```python
from build123d import *
from build123d.topology import SkipClean

# Parameters (mm, degrees)
EXTRUDE_2_DEPTH        = 8
SKETCH_5_W             = 850
SKETCH_5_H             = 100
EXTRUDE_3_DEPTH        = 8
SKETCH_6_W             = 850
SKETCH_6_H             = 8
EXTRUDE_4_DEPTH        = 84
SKETCH_7_R             = 13
CUT_EXTRUDE_1_DEPTH    = 905.579460302
SKETCH_9_R             = 13
CUT_EXTRUDE_3_DEPTH    = 904.800863022
PATTERN_LINEAR_2_COUNT = 6
PATTERN_LINEAR_2_PITCH = 160
MIRROR_7_DEPTH         = 16
MIRROR_7_2_OUTLINE_R   = 13
MIRROR_7_2_DEPTH       = 8
MIRROR_START           = 8
MIRROR_7_3_OUTLINE_R   = 13
MIRROR_7_3_DEPTH       = 8
MIRROR_START_2         = 16
MIRROR_7_4_OUTLINE_W   = 850
MIRROR_7_4_OUTLINE_H   = 8
MIRROR_7_4_DEPTH       = 84


# Read off the part's stored shape, not the designer's step: 镜向7
with BuildPart() as part:
    # 草图1 → 凸台-拉伸2 (new body)
    with BuildSketch(Plane.XY):
        Polygon((-870, 0), (-870, 230), (-770, 230), (0, 100), (0, 0), align=None)
    extrude_2 = extrude(amount=EXTRUDE_2_DEPTH)

    # 镜向2: 凸台-拉伸2 across plane
    add(extrude_2.mirror(Plane.ZX))

    # 草图5 → 凸台-拉伸3 (add)
    with BuildSketch(Plane.XY.offset(8)):
        with Locations((-425, 10)):
            Rectangle(SKETCH_5_W, SKETCH_5_H)
    extrude(amount=EXTRUDE_3_DEPTH)

    # 草图6 → 凸台-拉伸4 (add)
    with BuildSketch(Plane.XY.offset(16)):
        with Locations((-425, 56)):
            Rectangle(SKETCH_6_W, SKETCH_6_H)
    extrude(amount=EXTRUDE_4_DEPTH)

    # 草图7 → 切除-拉伸1 (cut, through all)
    with BuildSketch(Plane.XY.offset(8)):
        with Locations((-770.885465198, 130.885465198)):
            Circle(SKETCH_7_R)
        with Locations((-827.454007693, 187.454007693)):
            Circle(SKETCH_7_R)
    cut_extrude_1 = extrude(amount=-CUT_EXTRUDE_1_DEPTH, mode=Mode.SUBTRACT)

    # 镜向5: 切除-拉伸1 across plane
    add(cut_extrude_1.mirror(Plane.ZX), mode=Mode.SUBTRACT)

    # 草图9 → 切除-拉伸3 (cut, through all)
    with BuildSketch(Plane.XY.offset(16)):
        with Locations((-799.964208957, 0)):
            Circle(SKETCH_9_R)
    cut_extrude_3 = extrude(amount=-CUT_EXTRUDE_3_DEPTH, mode=Mode.SUBTRACT)

    # 阵列(线性)2: 切除-拉伸3 ×6
    with Locations(*[(i * PATTERN_LINEAR_2_PITCH, 0, 0) for i in range(1, PATTERN_LINEAR_2_COUNT)]):
        add(cut_extrude_3, mode=Mode.SUBTRACT)

    # 镜向7 outline → 镜向7 (cut)
    with BuildSketch(Plane.XY):
        with BuildLine():
            ThreePointArc((0, -12.999950731), (-12.964208957, 0), (0, 12.999950731))
            ThreePointArc((0, 12.999950731), (-13.035791043, 0), (0, -12.999950731))
        make_face()
    extrude(amount=MIRROR_7_DEPTH, mode=Mode.SUBTRACT)

    # Mirror 7 2 outline → Mirror 7 2 (add)
    with BuildSketch(Plane.XY):
        with BuildLine():
            Line((870, -230), (870, 230))
            Line((870, 230), (770, 230))
            Line((770, 230), (0, 100))
            Line((0, 100), (0, 12.999950731))
            ThreePointArc((0, 12.999950731), (12.964208957, 0), (0, -12.999950731))
            Line((0, -12.999950731), (0, -100))
            Line((0, -100), (770, -230))
            Line((770, -230), (870, -230))
        make_face()
        with Locations((827.454007693, -187.454007693)):
            Circle(MIRROR_7_2_OUTLINE_R, mode=Mode.SUBTRACT)
        with Locations((770.885465198, -130.885465198)):
            Circle(MIRROR_7_2_OUTLINE_R, mode=Mode.SUBTRACT)
        with Locations((770.885465198, 130.885465198)):
            Circle(MIRROR_7_2_OUTLINE_R, mode=Mode.SUBTRACT)
        with Locations((827.454007693, 187.454007693)):
            Circle(MIRROR_7_2_OUTLINE_R, mode=Mode.SUBTRACT)
        with Locations((639.964208957, 0)):
            Circle(MIRROR_7_2_OUTLINE_R, mode=Mode.SUBTRACT)
        with Locations((799.964208957, 0)):
            Circle(MIRROR_7_2_OUTLINE_R, mode=Mode.SUBTRACT)
        with Locations((159.964208957, 0)):
            Circle(MIRROR_7_2_OUTLINE_R, mode=Mode.SUBTRACT)
        with Locations((319.964208957, 0)):
            Circle(MIRROR_7_2_OUTLINE_R, mode=Mode.SUBTRACT)
        with Locations((479.964208957, 0)):
            Circle(MIRROR_7_2_OUTLINE_R, mode=Mode.SUBTRACT)
    extrude(amount=MIRROR_7_2_DEPTH)

    # Mirror 7 3 outline → Mirror 7 3 (add)
    with SkipClean():  # the faces are left unmerged after this step: merging them gives an invalid solid
        with BuildSketch(Plane.XY.offset(MIRROR_START)):
            with BuildLine():
                Line((850, 60), (0, 60))
                Line((0, 60), (0, 12.999950731))
                ThreePointArc((0, 12.999950731), (12.964208957, 0), (0, -12.999950731))
                Line((0, -12.999950731), (0, -40))
                Line((0, -40), (850, -40))
                Line((850, -40), (850, 60))
            make_face()
            with Locations((799.964208957, 0)):
                Circle(MIRROR_7_3_OUTLINE_R, mode=Mode.SUBTRACT)
            with Locations((159.964208957, 0)):
                Circle(MIRROR_7_3_OUTLINE_R, mode=Mode.SUBTRACT)
            with Locations((319.964208957, 0)):
                Circle(MIRROR_7_3_OUTLINE_R, mode=Mode.SUBTRACT)
            with Locations((479.964208957, 0)):
                Circle(MIRROR_7_3_OUTLINE_R, mode=Mode.SUBTRACT)
            with Locations((639.964208957, 0)):
                Circle(MIRROR_7_3_OUTLINE_R, mode=Mode.SUBTRACT)
        extrude(amount=MIRROR_7_3_DEPTH)

    # Mirror 7 4 outline → Mirror 7 4 (add)
    with SkipClean():  # the faces are left unmerged after this step: merging them gives an invalid solid
        with BuildSketch(Plane.XY.offset(MIRROR_START_2)):
            with Locations((425, 56)):
                Rectangle(MIRROR_7_4_OUTLINE_W, MIRROR_7_4_OUTLINE_H)
        extrude(amount=MIRROR_7_4_DEPTH)


solid = part.part
```
Design review of the part built by this model. Coordinates are the model's own, in mm. A direction names the side the tool comes from. Coordinates: 2 decimals unless noted, no trailing zeros. Order: outer loops, then holes, each group sorted by start corner. A loop starts at its lowest first (then second) coordinate and runs counter-clockwise, first axis right, second up. Notation, with made-up numbers: M -33,18.25 L 23,18.25 A17 cw 23,41.25 Z; hole C 28.25,-23 d2. An arc over 180 degrees is marked long. Answer as a JSON object with one key per item and string values. Group by question number.
1) Add section B-B, the plane x = -198.5. Write out the cut boundary in (y, z).
2) Add section C-C, the plane z = 72.5. Write out the cut boundary in (x, y).
3) Wall thickness on L1, parallel to Z at x = -798.5, y = -142; L2, parallel to Y at x = -574, z = 56.5; L3, parallel to Z at x = 269.5, y = 9.5: over which ranges is each line inside the solid? List them lowest first.
4) For pin 1 (10 mm diameter, centred on x = 24.5, z = 62.5, fed in from -Y); pin 2 (1.5 mm diameter, centred on x = 550, y = -92.5, fed in from +Z), all flat-tipped, find the tip position at first contact; note any pin that passes through.
5) Add section A-A, the plane y = 34.5. Write out the cut boundary in (x, z).
6) Tool access review of faces 1 (the flat face through (-12, 52, 57)), 2 (the flat face through (-390.39, 165.91, 3.94)), 3 (the flat face through (379.61, -164.09, 3.94)): name each direction out of +Z, -Z, +X, -X, +Y, -Y from which nothing blocks a thin tool from reaching the whole face with its end or side.
Computed values:
{
 "1": {"outline": "M -133.51,0 L 133.51,0 L 133.51,8 L 60,8 L 60,100 L 52,100 L 52,16 L -40,16 L -40,8 L -133.51,8 Z"},
 "2": {"outline": "M -850,52 L 850,52 L 850,60 L -850,60 Z"},
 "3": {"L1": "z = 0 to 8", "L2": "y = 52 to 60", "L3": "z = 0 to 16"},
 "4": {"pin 1": "stops at y = 52", "pin 2": "stops at z = 8"},
 "5": {"outline": "M -870,0 L 870,0 L 870,8 L 850,8 L 850,16 L -850,16 L -850,8 L -870,8 Z"},
 "6": {"face 1": "+Z, +X, -X, -Y", "face 2": "+Z, -Z, +Y", "face 3": "+Z, -Z, -Y"}
}
